Can you work these out from the model? Positions are in its coordinate system, mm. Round coordinates to 2 decimals unless told otherwise and drop trailing zeros. Write each loop counter-clockwise with the first axis right and the second up, starting at its lowest first coordinate (ties: lowest second). Pieces come first, ordered by that corner, then holes. Notation, with made-up numbers: (25, -23.5) -> (79, -23.5) arc R33 ccw to (79, 4.5) -> close; hole circle Ø3 at (-14, 62.25). An arc over 180 degrees is marked (long way). Write item = value, one per line. Start each with the question number.
1) Imagine slicing it at B-B, the plane x = -1.75. Please give me the cut outline in (y, z).
2) Thinking about a two-plate mould opening in Y: for faces 1 (the face through (-4, -2, 0)), 2 (the face through (-4.76, 0.39, 0.15)), which applies, +Y half, -Y half, draft (parallel to the pull), parting line (faces both ways), or undercut?
3) If I drill on line 1 (X direction, y = 1, z = 0.05); line 2 (X direction, y = 5.5, z = 0.15); line 3 (Y direction, x = 6, z = 0.1), over which ranges is the centre line in solid material (lowest first)?
4) Imagine slicing it at D-D, the plane y = 1. Please give me the cut outline in (x, z), then the cut area to 3 significant figures.
5) Imagine slicing it at C-C, the plane y = 5.75. Please give me the cut outline in (x, z), then the cut area to 3 significant figures.
6) Imagine slicing it at A-A, the plane z = 0.15. Please give me the cut outline in (x, y), then the cut area to 3 significant figures.
from build123d import *

# Parameters (mm, degrees)
F0_R     = 8.05
F0_R_2   = 1.3
F1_DEPTH = 0.3


with BuildPart() as f1:
    # F0 (on Top) → F1 (new body)
    with BuildSketch(Plane.XY):
        Circle(F0_R)
        with BuildLine():
            ThreePointArc((1.3, -6), (-0.919239, -6.919239), (0, -4.7))
            ThreePointArc((0, -4.7), (0.919239, -5.080761), (1.3, -6))
        make_face(mode=Mode.SUBTRACT)
        with Locations((-6, 0)):
            Circle(F0_R_2, mode=Mode.SUBTRACT)
        with BuildLine():
            ThreePointArc((0, -3.95), (-2.793072, -2.793072), (-3.95, 0))
            ThreePointArc((-3.95, 0), (-2.793072, 2.793072), (0, 3.95))
            ThreePointArc((0, 3.95), (2.793072, 2.793072), (3.95, 0))
            ThreePointArc((3.95, 0), (2.793072, -2.793072), (0, -3.95))
        make_face(mode=Mode.SUBTRACT)
        with BuildLine():
            ThreePointArc((7.3, 0), (6, -1.3), (4.7, 0))
            ThreePointArc((4.7, 0), (6, 1.3), (7.3, 0))
        make_face(mode=Mode.SUBTRACT)
        with BuildLine():
            ThreePointArc((1.3, 6), (0.919239, 5.080761), (0, 4.7))
            ThreePointArc((0, 4.7), (-0.919239, 6.919239), (1.3, 6))
        make_face(mode=Mode.SUBTRACT)
    extrude(amount=F1_DEPTH)


solid = f1.part
Reported:
q1.outline = (-7.86, 0) -> (-3.54, 0) -> (-3.54, 0.3) -> (-7.86, 0.3) -> close; (3.54, 0) -> (7.86, 0) -> (7.86, 0.3) -> (3.54, 0.3) -> close
q2.face_1 = draft
q2.face_2 = undercut
q3.line_1 = -7.99 to -6.83, -5.17 to -3.82, 3.82 to 5.17, 6.83 to 7.99
q3.line_2 = -5.88 to -1.2, 1.2 to 5.88
q3.line_3 = -5.37 to -1.3, 1.3 to 5.37
q4.outline = (-7.99, 0) -> (-6.83, 0) -> (-6.83, 0.3) -> (-7.99, 0.3) -> close; (-5.17, 0) -> (-3.82, 0) -> (-3.82, 0.3) -> (-5.17, 0.3) -> close; (3.82, 0) -> (5.17, 0) -> (5.17, 0.3) -> (3.82, 0.3) -> close; (6.83, 0) -> (7.99, 0) -> (7.99, 0.3) -> (6.83, 0.3) -> close
q4.area = 1.50 mm²
q5.outline = (-5.63, 0) -> (-1.28, 0) -> (-1.28, 0.3) -> (-5.63, 0.3) -> close; (1.28, 0) -> (5.63, 0) -> (5.63, 0.3) -> (1.28, 0.3) -> close
q5.area = 2.61 mm²
q6.outline = circle Ø16.1 at (0, 0); hole circle Ø2.6 at (-6, 0); hole (-3.95, 0) arc R3.95 ccw to (0, -3.95) arc R3.95 ccw to (3.95, 0) arc R3.95 ccw to (0, 3.95) arc R3.95 ccw to start; hole circle Ø2.6 at (0, -6); hole circle Ø2.6 at (0, 6); hole circle Ø2.6 at (6, 0)
q6.area = 133 mm²
